```python
from build123d import *

# Parameters (mm, degrees)
SKETCH_1_R          = 1.5
EXTRUDE_1_DEPTH     = 3
SKETCH_2_W          = 20
SKETCH_2_H          = 3
SKETCH_2_W_2        = 7
SKETCH_2_W_3        = 6
CUT_EXTRUDE_1_DEPTH = 3


with BuildPart() as part:
    # 草图1 → 凸台-拉伸1 (new body)
    with BuildSketch(Plane(origin=(0, 0, 0), x_dir=(1, 0, 0), z_dir=(0, 1, 0))):
        Polygon((-3, 36), (3, 36), (3, 33), (10, 33), (10, 36), (30, 36), (30, -36), (10, -36), (10, -33), (3, -33), (3, -36), (-3, -36), (-3, -33), (-10, -33), (-10, -36), (-30, -36), (-30, 36), (-10, 36), (-10, 33), (-3, 33), align=None)
        with Locations(Location((-20, 0, 0), (0, 0, 270))):
            Circle(SKETCH_1_R, mode=Mode.SUBTRACT)
        with Locations(Location((-20, 10, 0), (0, 0, 270))):
            Circle(SKETCH_1_R, mode=Mode.SUBTRACT)
        with Locations(Location((-20, -10, 0), (0, 0, 270))):
            Circle(SKETCH_1_R, mode=Mode.SUBTRACT)
        with Locations(Location((20, -10, 0), (0, 0, 90))):
            Circle(SKETCH_1_R, mode=Mode.SUBTRACT)
        with Locations(Location((20, 0, 0), (0, 0, 90))):
            Circle(SKETCH_1_R, mode=Mode.SUBTRACT)
        with Locations(Location((20, 10, 0), (0, 0, 90))):
            Circle(SKETCH_1_R, mode=Mode.SUBTRACT)
    extrude(amount=EXTRUDE_1_DEPTH)

    # 草图2 → 切除-拉伸1 (cut)
    with BuildSketch(Plane(origin=(0, 3, 0), x_dir=(1, 0, 0), z_dir=(0, 1, 0))):
        Polygon((10, -36), (10, -33), (3, -33), (3, -36), (-3, -36), (-3, -33), (-10, -33), (-10, -36), (-30, -36), (-30, -51.145267559), (30, -51.145267559), (30, -36), align=None)
        with Locations((20, -34.5)):
            Rectangle(SKETCH_2_W, SKETCH_2_H)
        with Locations((6.5, -31.5)):
            Rectangle(SKETCH_2_W_2, SKETCH_2_H)
        with Locations((0, -34.5)):
            Rectangle(SKETCH_2_W_3, SKETCH_2_H)
        with Locations((-6.5, -31.5)):
            Rectangle(SKETCH_2_W_2, SKETCH_2_H)
        with Locations((-20, -34.5)):
            Rectangle(SKETCH_2_W, SKETCH_2_H)
        with Locations((-20, 34.5)):
            Rectangle(SKETCH_2_W, SKETCH_2_H)
        with Locations((-6.5, 31.5)):
            Rectangle(SKETCH_2_W_2, SKETCH_2_H)
        with Locations((0, 34.5)):
            Rectangle(SKETCH_2_W_3, SKETCH_2_H)
        with Locations((6.5, 31.5)):
            Rectangle(SKETCH_2_W_2, SKETCH_2_H)
        with Locations((20, 34.5)):
            Rectangle(SKETCH_2_W, SKETCH_2_H)
    extrude(amount=-CUT_EXTRUDE_1_DEPTH, mode=Mode.SUBTRACT)


solid = part.part
```
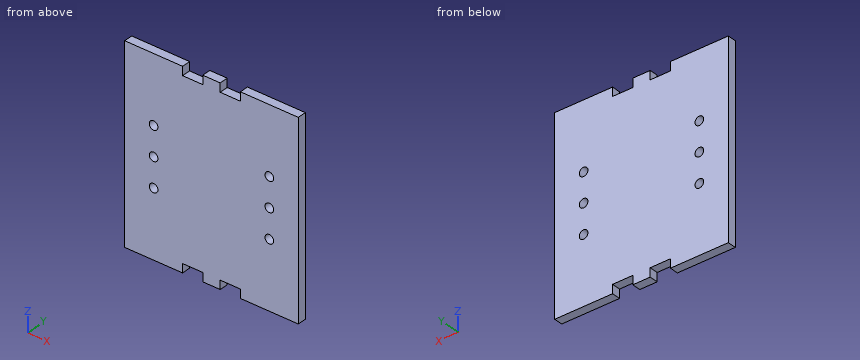
Geometry check sheet. Reference: the model listing, model coordinates, mm. Coordinates: 2 decimals unless noted, no trailing zeros. Write each loop counter-clockwise with the first axis right and the second up, starting at its lowest first coordinate (ties: lowest second). Pieces come first, ordered by that corner, then holes. Notation, with made-up numbers: M -39.5,27.5 L -13.5,27.5 A17 ccw -13.5,46.5 Z; hole C 34,16 d8. An arc over 180 degrees is marked long. One line per item, written item: value. Start each with the question number.
(1) Sectioned sample at D-D, the plane x = -4.5. Enter the section's corners in (y, z).
(2) Depth check by flat-ended pin: pin 1 (4 mm diameter, centred on x = -20, z = -10, fed in from +Y); pin 2 (1.5 mm diameter, centred on x = 5.5, y = 1, fed in from +Z); pin 3 (2.5 mm diameter, centred on x = -20, z = 10, fed in from +Y). Enter the tip coordinate at first touch or a pass-through.
(3) Sectioned sample at B-B, the plane z = -10. Enter the section's corners in (x, y), and give its area (3 significant figures).
(4) Sectioned sample at A-A, the plane x = -20. Enter the section's corners in (y, z).
(5) Sectioned sample at C-C, the plane y = 1.6. Enter the section's corners in (x, z), and give its area (3 significant figures).
(6) Scan lines: line 1 along X through (y, z) = (2.05, 0); line 2 along X through (y, z) = (1.7, 30.5); line 3 along Z through (x, y) = (21, 1.65). Record each from-to range of solid material in increasing order. Write a range as [from, to].
Filled sheet:
1. outline: M 0,-30 L 3,-30 L 3,30 L 0,30 Z
2. pin 1: y = 3
2. pin 2: z = 30
2. pin 3: through
3. outline: M -30,0 L -21.5,0 L -21.5,3 L -30,3 Z; M -18.5,0 L 18.5,0 L 18.5,3 L -18.5,3 Z; M 21.5,0 L 30,0 L 30,3 L 21.5,3 Z
3. area: 162 mm²
4. outline: M 0,-33 L 3,-33 L 3,-11.5 L 0,-11.5 Z; M 0,-8.5 L 3,-8.5 L 3,-1.5 L 0,-1.5 Z; M 0,1.5 L 3,1.5 L 3,8.5 L 0,8.5 Z; M 0,11.5 L 3,11.5 L 3,33 L 0,33 Z
5. outline: M -30,-33 L -10,-33 L -10,-30 L -3,-30 L -3,-33 L 3,-33 L 3,-30 L 10,-30 L 10,-33 L 30,-33 L 30,33 L 10,33 L 10,30 L 3,30 L 3,33 L -3,33 L -3,30 L -10,30 L -10,33 L -30,33 Z; hole C -20,-10 d3; hole C -20,0 d3; hole C -20,10 d3; hole C 20,-10 d3; hole C 20,0 d3; hole C 20,10 d3
5. area: 3,830 mm²
6. line 1: [-30, -21.5], [-18.5, 18.5], [21.5, 30]
6. line 2: [-30, -10], [-3, 3], [10, 30]
6. line 3: [-33, -11.12], [-8.88, -1.12], [1.12, 8.88], [11.12, 33]
